```python
from build123d import *

# Parameters (mm, degrees)
SKETCH1_R               = 2.38125
BOSS_EXTRUDE1_DEPTH     = 5.588
CUT_EXTRUDE2_DEPTH      = 15.583449318
CUT_EXTRUDE2_DEPTH_BACK = 15.583449318
SKETCH2_R               = 0.5


with BuildPart() as part:
    # Sketch1 → Boss-Extrude1 (new body)
    with BuildSketch(Plane.XY):
        Polygon((-2.794, 3.175), (-2.794, 9.525), (-9.525, 9.525), (-9.525, -9.525), (-2.794, -9.525), (-2.794, -3.175), (2.794, -3.175), (2.794, -9.525), (9.525, -9.525), (9.525, 9.525), (2.794, 9.525), (2.794, 3.175), align=None)
        Circle(SKETCH1_R, mode=Mode.SUBTRACT)
    extrude(amount=BOSS_EXTRUDE1_DEPTH)

    # Sketch2 → Cut-Extrude2 (cut, two sides: drawn at the far end of the back side and taken through both)
    with BuildSketch(Plane.XY.offset(-CUT_EXTRUDE2_DEPTH_BACK)):
        with Locations((-2.794, 3.175)):
            Circle(SKETCH2_R)
        with Locations((2.794, 3.175)):
            Circle(SKETCH2_R)
        with Locations((2.794, -3.175)):
            Circle(SKETCH2_R)
        with Locations((-2.794, -3.175)):
            Circle(SKETCH2_R)
    extrude(amount=CUT_EXTRUDE2_DEPTH + CUT_EXTRUDE2_DEPTH_BACK, mode=Mode.SUBTRACT)


solid = part.part
```
Geometry: final body of the model. Coordinates: model frame, mm. A direction names the side the tool comes from. Round coordinates to 2 decimals unless told otherwise and drop trailing zeros. Loops run counter-clockwise (first coordinate to the right, second up) from the corner with the lowest first, then second, coordinate; pieces in that order, holes last.
Item 1: Section B-B, the plane x = 0. Output: boundary loops of the cut face in (y, z) (3 decimals), plus the area to 3 significant figures.
Checked values:
outline: (-3.175, 0) - (-2.381, 0) - (-2.381, 5.588) - (-3.175, 5.588) - close; (2.381, 0) - (3.175, 0) - (3.175, 5.588) - (2.381, 5.588) - close
area: 8.87 mm2
Item 2: Section C-C, the plane z = 2.45. Output: boundary loops of the cut face in (x, y) (1 decimal), plus the area to 3 significant figures.
Checked values:
outline: (-9.5, -9.5) - (-2.8, -9.5) - (-2.8, -3.7) arc R0.5 cw (long way) to (-2.3, -3.2) - (2.3, -3.2) arc R0.5 cw (long way) to (2.8, -3.7) - (2.8, -9.5) - (9.5, -9.5) - (9.5, 9.5) - (2.8, 9.5) - (2.8, 3.7) arc R0.5 cw (long way) to (2.3, 3.2) - (-2.3, 3.2) arc R0.5 cw (long way) to (-2.8, 3.7) - (-2.8, 9.5) - (-9.5, 9.5) - close; hole circle Ø4.8 at (0, 0)
area: 272 mm2
Item 3: Reachability of faces 5 (the flat face through (-2.794, 7, 3)), 6 (the flat face through (0, -3.175, 3)), 7 (the cylindrical face through (3.159, -2.833, 2.755)) from +Z, -Z, +X, -X, +Y, -Y: full face, straight path, thin tool, end or side. Return the list, or none.
Checked values:
face 5: +Z, -Z, +Y
face 6: +Z, -Z, -Y
face 7: +Z, -Z
Item 4: Section A-A, the plane y = -8.5. Output: boundary loops of the cut face in (x, z) (3 decimals), plus the area to 3 significant figures.
Checked values:
outline: (-9.525, 0) - (-2.794, 0) - (-2.794, 5.588) - (-9.525, 5.588) - close; (2.794, 0) - (9.525, 0) - (9.525, 5.588) - (2.794, 5.588) - close
area: 75.2 mm2
Item 5: Mould query, pull axis Y, two halves, no side actions, for faces 1 (the cylindrical face through (-3.136, -2.81, 2.755)), 2 (the cylindrical face through (-1.89, -1.45, 2.75)), 3 (the flat face through (2, 2, 0)), 4 (the flat face through (-6, -9.525, 3)). Classes: released by +Y, released by -Y, zero draft, split by the parting line, or undercut.
Checked values:
face 1: undercut
face 2: undercut
face 3: zero draft
face 4: released by -Y
Item 6: Line query: L1, parallel to X at y = 6.75, z = 2.7 (3 decimals); L2, parallel to Y at x = 0, z = 2.8 (3 decimals); L3, parallel to X at y = 0.25, z = 3.1 (3 decimals). Output: solid intervals per line, ascending.
Checked values:
L1: x = -9.525 to -2.794, 2.794 to 9.525
L2: y = -3.175 to -2.381, 2.381 to 3.175
L3: x = -9.525 to -2.368, 2.368 to 9.525
